Autodesk Inventor part; units mm, degrees
ref_plane "YZ Plane" through (0, 0, 0) normal (1, 0, 0) x (0, 1, 0)
ref_plane "XZ Plane" through (0, 0, 0) normal (0, 1, 0) x (-1, 0, 0)
ref_plane "XY Plane" through (0, 0, 0) normal (0, 0, 1) x (1, 0, 0)
sketch "Sketch1" plane through (0, 0, 0) normal (0, 0, 1) x (1, 0, 0)
  line L0 (0, 0) -> (144, 0)
  line L1 (144, 0) -> (144, 77)
  line L2 (144, 77) -> (0, 77)
  line L3 (0, 77) -> (0, 0)
  dimension "d0" = 144
  dimension "d1" = 77
extrude "Extrusion1" add sketch "Sketch1" along normal blind 3
sketch "Sketch2" plane through (0, 0, 3) normal (0, 0, 1) x (1, 0, 0)
  line L0 (144, 77) -> (0, 77)
  line L1 (0, 0) -> (144, 0)
  line L2 (0, 77) -> (144, 77)
  line L3 (144, 77) -> (144, 0)
  line L4 (144, 0) -> (0, 0)
  line L5 (0, 0) -> (0, 77)
  line L6 (7, 0) -> (7, -3)
  line L7 (7, -3) -> (17, -3)
  line L8 (17, -3) -> (17, 0)
  line L9 (27, 0) -> (27, -3)
  line L10 (27, -3) -> (37, -3)
  line L11 (37, -3) -> (37, 0)
  line L12 (47, 0) -> (47, -3)
  line L13 (47, -3) -> (57, -3)
  line L14 (57, -3) -> (57, 0)
  line L15 (67, 0) -> (67, -3)
  line L16 (67, -3) -> (77, -3)
  line L17 (77, -3) -> (77, 0)
  line L18 (87, 0) -> (87, -3)
  line L19 (87, -3) -> (97, -3)
  line L20 (97, -3) -> (97, 0)
  line L21 (107, 0) -> (107, -3)
  line L22 (107, -3) -> (117, -3)
  line L23 (117, -3) -> (117, 0)
  line L24 (127, 0) -> (127, -3)
  line L25 (127, -3) -> (137, -3)
  line L26 (137, -3) -> (137, 0)
  line L27 (0, 77) -> (0, 0)
  line L28 (0, 10) -> (-3, 10)
  line L29 (-3, 10) -> (-3, 20)
  line L30 (-3, 20) -> (0, 20)
  line L31 (-3, 40) -> (0, 40)
  line L32 (-3, 30) -> (-3, 40)
  line L33 (0, 30) -> (-3, 30)
  line L34 (-3, 60) -> (0, 60)
  line L35 (-3, 50) -> (-3, 60)
  line L36 (0, 50) -> (-3, 50)
  line L37 (144, 77) -> (0, 77)
  line L38 (0, 77) -> (-3, 77)
  line L39 (-3, 77) -> (-3, 70)
  line L40 (-3, 70) -> (0, 70)
  line L41 (144, 0) -> (144, 77)
  line L42 (144, 77) -> (147, 77)
  line L43 (147, 77) -> (147, 70)
  line L44 (147, 70) -> (144, 70)
  line L45 (144, 0) -> (144, 77)
  line L46 (144, 60) -> (147, 60)
  line L47 (147, 60) -> (147, 50)
  line L48 (147, 50) -> (144, 50)
  line L49 (144, 40) -> (147, 40)
  line L50 (147, 40) -> (147, 30)
  line L51 (147, 30) -> (144, 30)
  line L52 (144, 20) -> (147, 20)
  line L53 (147, 20) -> (147, 10)
  line L54 (147, 10) -> (144, 10)
  dimension "d11" = 10
  dimension "d4" = 3
  dimension "d5" = 10
  dimension "d8" = 20
  dimension "d13" = 3
  dimension "d14" = 10
  dimension "d17" = 20
  dimension "d22" = 3
  dimension "d23" = 7
  dimension "d24" = 3
extrude "Extrusion2" add sketch "Sketch2" against normal blind 3 contours L42 L43 L44 L3 | L5 L40 L39 L38 | L46 L47 L48 L3 | L5 L36 L35 L34 | L49 L50 L51 L3 | L5 L33 L32 L31 | L52 L53 L54 L3 | L5 L28 L29 L30 | L26 L25 L24 L1 | L1 L8 L7 L6 | L23 L22 L21 L1 | L1 L11 L10 L9 | L20 L19 L18 L1 | L1 L14 L13 L12 | L17 L16 L15 L1
sketch "Sketch3" plane through (0, 0, 3) normal (0, 0, 1) x (1, 0, 0)
  line L0 (0, 74) -> (7, 74)
  line L1 (7, 74) -> (7, 71)
  line L2 (7, 71) -> (0, 71)
  line L3 (0, 71) -> (0, 74)
  line L4 (137, 74) -> (144, 74)
  line L5 (144, 74) -> (144, 71)
  line L6 (144, 71) -> (137, 71)
  line L7 (137, 71) -> (137, 74)
  line L8 (0, 36) -> (7, 36)
  line L9 (7, 36) -> (7, 33)
  line L10 (7, 33) -> (0, 33)
  line L11 (0, 33) -> (0, 36)
  line L12 (137, 36) -> (144, 36)
  line L13 (144, 36) -> (144, 33)
  line L14 (144, 33) -> (137, 33)
  line L15 (137, 33) -> (137, 36)
  line L16 (7, 30) -> (7, 27)
  line L17 (7, 27) -> (0, 27)
  line L18 (0, 27) -> (0, 30)
  line L19 (0, 30) -> (7, 30)
  line L20 (144, 36) -> (144, 33)
  line L21 (144, 33) -> (137, 33)
  line L22 (137, 33) -> (137, 36)
  line L23 (137, 36) -> (144, 36)
  line L24 (144, 30) -> (144, 27)
  line L25 (144, 27) -> (137, 27)
  line L26 (137, 27) -> (137, 30)
  line L27 (137, 30) -> (144, 30)
  point P0 (0, 0)
  dimension "d27" = 7
  dimension "d28" = 3
  dimension "d31" = 137
  dimension "d34" = 38
  dimension "d41" = 6
  dimension "d44" = 137
extrude "Extrusion3" cut sketch "Sketch3" against normal through all
properties part number "DoosjeVoorkant" material "Wood (Cherry)"
Can you work these out from the model? Positions are in its coordinate system, mm. A direction names the side the tool comes from. Give positions to 0.01 mm unless a question says otherwise; leave off trailing zeros. Loops run counter-clockwise (first coordinate to the right, second up) from the corner with the lowest first, then second, coordinate; pieces in that order, holes last. Notation, with made-up numbers: M 30.25,4.5 L 40.25,4.5 A31 cw 40.25,38.5 Z; hole C 57,-33 d11. An arc over 180 degrees is marked long. One line per item, written item: value.
(1) Suppose I cut it at C-C on x = 65.5. List the corners of the cut face in (y, z) for me, plus the area to 3 significant figures.
Returned:
outline: M 0,0 L 77,0 L 77,3 L 0,3 Z
area: 231 mm^2
(2) Suppose I cut it at B-B on y = 6. List the corners of the cut face in (x, z) for me, plus the area to 3 significant figures.
Returned:
outline: M 0,0 L 144,0 L 144,3 L 0,3 Z
area: 432 mm^2
(3) Which directions (+Z, -Z, +X, -X, +Y, -Y) give clear straight access to the entire face, cutting with the end or side of a thin tool? Please do faces 4 (the face through (141, 33, 2)), 5 (the face through (2, 30, 2)), 6 (the face through (122, 0, 1)), 7 (the face through (144, 65, 1)).
Returned:
face 4: +Z, -Z
face 5: +Z, -Z, -X
face 6: +Z, -Z, -Y
face 7: +Z, -Z, +X
(4) I need wall thicknesses on line 1 (Y direction, x = 5.5, z = 0.45); line 2 (Y direction, x = 60.5, z = 1.9); line 3 (X direction, y = 3, z = 2.9). Which ranges of each line are inside material? Lowest first, please.
Returned:
line 1: 0 to 27, 30 to 33, 36 to 71, 74 to 77
line 2: 0 to 77
line 3: 0 to 144
(5) Will these pins go through, and if not, where does the flat tip stop? pin 1 (0.9 mm diameter, centred on x = 145, z = 1.5, fed in from -Y); pin 2 (0.9 mm diameter, centred on x = 2, z = 1, fed in from -Y); pin 3 (0.9 mm diameter, centred on y = -1.5, z = 1, fed in from +X).
Returned:
pin 1: y = 10
pin 2: y = 0
pin 3: x = 137
(6) Suppose I cut it at A-A on z = 2.4. Count the separate pieces of the cut face and the enclosed holes in it, plus the area to 3 significant figures.
Returned:
separate pieces: 1
enclosed holes: 4
area: 11,400 mm^2
(7) We'd pull the mould along X, two halves only. Please class faces 1 (the face through (3, 36, 2)), 2 (the face through (112, -3, 2)), 3 (the face through (147, 35, 2)): released by +X, released by -X, zero draft, split by the parting line, or undercut.
Returned:
face 1: undercut
face 2: zero draft
face 3: released by +X
